Autodesk Inventor part; units mm, degrees
ref_plane "Work Plane1" through (0, 0, 9.75) normal (0, 0, 1) x (1, 0, 0)
ref_plane "YZ Plane" through (0, 0, 0) normal (1, 0, 0) x (0, 1, 0)
ref_plane "XZ Plane" through (0, 0, 0) normal (0, 1, 0) x (-1, 0, 0)
sketch "Sketch1" plane through (0, 0, 0) normal (0, 0, 1) x (1, 0, 0)
  circle A0 centre (0, 0) radius 6
  line L0 (-10, -12.75) -> (10, -12.75)
  line L1 (10, -12.75) -> (10, 12.75)
  line L2 (10, 12.75) -> (-10, 12.75)
  line L3 (-10, 12.75) -> (-10, -12.75)
  line L4 (-10, -12.75) -> (10, 12.75) construction
  line L5 (10, -12.75) -> (-10, 12.75) construction
  line L6 (-10, -12.75) -> (-21, -12.75)
  line L7 (-21, -12.75) -> (-21, 12.75)
  line L8 (-21, 12.75) -> (-10, 12.75)
  line L9 (-10, 12.75) -> (-10, -12.75)
  dimension "d0" = 12
  dimension "d1" = 25.5
  dimension "d2" = 20
  dimension "d20" = 11
extrude "Extrusion1" add sketch "Sketch1" along normal blind 19.5 contours A0 | L3 L2 L1 L0 | L6 L7 L8 L3
ref_plane "Work Plane1" through (0, 0, 9.75) normal (0, 0, 1) x (1, 0, 0)
sketch "Sketch2" plane through (0, 0, 9.75) normal (0, 0, 1) x (1, 0, 0)
  circle A0 centre (0, 0) radius 9.5
  line L0 (-10, -9.5) -> (10, -9.5)
  line L1 (10, -9.5) -> (10, 9.5)
  line L2 (10, 9.5) -> (-10, 9.5)
  line L3 (-10, 9.5) -> (-10, -9.5)
  line L4 (-10, -9.5) -> (10, 9.5) construction
  line L5 (10, -9.5) -> (-10, 9.5) construction
  point P0 (0, 9.5)
  point P1 (0, -9.5)
  dimension "d5" = 19
  dimension "d6" = 20
  dimension "d7" = 19
extrude "Extrusion2" cut sketch "Sketch2" along normal mid plane 15 contours A0 | A0 L2 L1 L0
sketch "Sketch3" plane through (0, 0, 19.5) normal (0, 0, 1) x (1, 0, 0)
  point P0 (0, 0)
  point P1 (0, 0)
hole "Hole1" at (0, 0, 19.5) direction (0, 0, -1) diameter 5.5 end through all
sketch "Sketch4" plane through (-21, -12.75, 0) normal (-1, 0, 0) x (0, 0, 1)
  line L0 (0, 25.5) -> (19.5, 25.5)
  line L1 (9.75, 25.5) -> (9.75, 0)
  line L2 (0, 0) -> (19.5, 0)
  point P0 (9.75, 20.5)
  point P1 (9.75, 5)
  dimension "d21" = 5
  dimension "d22" = 5
hole "Hole2" at (-21, 7.75, 9.75) at (-21, -7.75, 9.75) direction (1, 0, 0) diameter 3.4 depth 8
sketch "Sketch5" plane through (0, 0, 19.5) normal (0, 0, 1) x (1, 0, 0)
  line L0 (-21, 6.05) -> (-21, 9.45)
  line L1 (-13, 9.45) -> (-13, 6.05)
  line L2 (-21, -9.45) -> (-21, -6.05)
  line L3 (-13, -6.05) -> (-13, -9.45)
  line L4 (-21, 7.75) -> (-13, 7.75)
  line L5 (-21, -7.75) -> (-13, -7.75)
  line L6 (-18.25, 10.5) -> (-15.75, 10.5)
  line L7 (-15.75, 10.5) -> (-15.75, 5)
  line L8 (-15.75, 5) -> (-18.25, 5)
  line L9 (-18.25, 5) -> (-18.25, 10.5)
  line L10 (-18.25, 10.5) -> (-15.75, 5) construction
  line L11 (-15.75, 10.5) -> (-18.25, 5) construction
  line L12 (-18.25, -5) -> (-15.75, -5)
  line L13 (-15.75, -5) -> (-15.75, -10.5)
  line L14 (-15.75, -10.5) -> (-18.25, -10.5)
  line L15 (-18.25, -10.5) -> (-18.25, -5)
  line L16 (-18.25, -5) -> (-15.75, -10.5) construction
  line L17 (-15.75, -5) -> (-18.25, -10.5) construction
  point P0 (0, 0)
  point P1 (-17, 7.75)
  point P2 (-17, -7.75)
  dimension "d30" = 2.5
  dimension "d31" = 5.5
  dimension "d32" = 2.5
  dimension "d33" = 5.5
extrude "Extrusion3" cut sketch "Sketch5" against normal blind 13
chamfer "Chamfer1" distance 2 angle 45 2 edges at (-15.75, 7.75, 19.5) (-15.75, -7.75, 19.5)
chamfer "Chamfer2" distance 0.5 angle 45 12 edges at (-21, 12.75, 9.75) (-21, 0, 0) (-21, -12.75, 9.75) (-21, 0, 19.5) (-5.5, 12.75, 19.5) (-5.5, 12.75, 0) (-5.5, -12.75, 0) (-5.5, -12.75, 19.5) (10, 0, 19.5) (10, 12.75, 9.75) (10, 0, 0) (10, -12.75, 9.75)
properties part number "X-End-Floating-Idler v0.1"
Check sheet for the modelled part. Datum: model origin and axes. Units: mm. A direction names the side the tool comes from. Give positions to 0.01 mm unless a question says otherwise; leave off trailing zeros. Loops run counter-clockwise (first coordinate to the right, second up) from the corner with the lowest first, then second, coordinate; pieces in that order, holes last. Notation, with made-up numbers: M -35,89 L -11,89 A27 ccw -11,107 Z; hole C 87.5,-23.5 d11. An arc over 180 degrees is marked long. Use a Markdown table: item, result. Add a question column.
Q1. Go/stop test with flat-tipped pins: pin 1 (0.8 mm diameter, centred on x = -17, y = 7, fed in from +Z); pin 2 (3 mm diameter, centred on y = -4.5, z = 9, fed in from +X); pin 3 (4 mm diameter, centred on y = -0.5, z = 13.5, fed in from +X). Record where each tip stops, or that it passes through.
Q2. Sectioned sample at D-D, the plane z = 7.5. Record the cut outline in (x, y).
Q3. Mould release check, pull along Y, two halves, no side actions. Record for faces 1 (the flat face through (10, 0, 18)), 2 (the flat face through (5, 9.5, 10)), 3 (the flat face through (-6, -12.75, 10)): pulls with the +Y half, pulls with the -Y half, needs draft (parallel to the pull), parting line crosses it, or undercut.
Q4. Sectioned sample at C-C, the plane z = 3. Record the cut outline in (x, y).
Q5. Sectioned sample at A-A, the plane y = 0. Record the cut outline in (x, z).
Q6. Tool access check on faces 4 (the flat face through (-14.76, 7.71, 18.49)), 5 (the cylindrical face through (-14.36, 9.41, 9.38)), 6 (the flat face through (5, -9.5, 10)). Record the directions out of +Z, -Z, +X, -X, +Y, -Y that give a thin tool (end or side, any length) a straight path to the whole face; none if there is none.
Q7. Scan lines: line 1 along Y through (x, z) = (-13.8, 9.75); line 2 along X through (y, z) = (-10.25, 8.5); line 3 along Y through (x, z) = (0, 18.8). Record each from-to range of solid material in increasing order. Write a range as [from, to].
Q8. Sectioned sample at B-B, the plane x = 7. Record the cut outline in (y, z).
Verdict:
| question | item | result |
|---|---|---|
| 1 | pin 1 | z = 6.5 |
| 1 | pin 2 | x = -7.37 |
| 1 | pin 3 | x = -9.17 |
| 2 | outline | M -21,-12.25 L -20.5,-12.75 L 9.5,-12.75 L 10,-12.25 L 10,-9.5 L 0,-9.5 A9.5 cw 0,9.5 L 10,9.5 L 10,12.25 L 9.5,12.75 L -20.5,12.75 L -21,12.25 Z; hole M -18.25,-10.5 L -15.75,-10.5 L -15.75,-5 L -18.25,-5 Z; hole M -18.25,5 L -15.75,5 L -15.75,10.5 L -18.25,10.5 Z |
| 3 | face 1 | needs draft |
| 3 | face 2 | undercut |
| 3 | face 3 | pulls with the -Y half |
| 4 | outline | M -21,-12.25 L -20.5,-12.75 L 9.5,-12.75 L 10,-12.25 L 10,-9.5 L 0,-9.5 A9.5 cw 0,9.5 L 10,9.5 L 10,12.25 L 9.5,12.75 L -20.5,12.75 L -21,12.25 Z |
| 5 | outline | M -21,0.5 L -20.5,0 L -2.75,0 L -2.75,2.25 L -9.5,2.25 L -9.5,17.25 L -2.75,17.25 L -2.75,19.5 L -20.5,19.5 L -21,19 Z; M 2.75,0 L 9.5,0 L 10,0.5 L 10,2.25 L 2.75,2.25 Z; M 2.75,17.25 L 10,17.25 L 10,19 L 9.5,19.5 L 2.75,19.5 Z |
| 6 | face 4 | +Z |
| 6 | face 5 | -X |
| 6 | face 6 | +X |
| 7 | line 1 | [-12.75, -9.45], [-6.05, 6.05], [9.45, 12.75] |
| 7 | line 2 | [-21, -18.25], [-15.75, 10] |
| 7 | line 3 | [-12.75, -2.75], [2.75, 12.75] |
| 8 | outline | M -12.75,0.5 L -12.25,0 L 12.25,0 L 12.75,0.5 L 12.75,19 L 12.25,19.5 L -12.25,19.5 L -12.75,19 Z; hole M -9.5,2.25 L 9.5,2.25 L 9.5,17.25 L -9.5,17.25 Z |
